The model under review builds one solid part; all positions refer to its coordinate system, in mm. Face numbers are marked on the shaded views. A direction names the side the tool comes from. Give positions to 0.01 mm unless a question says otherwise; leave off trailing zeros. Loops run counter-clockwise (first coordinate to the right, second up) from the corner with the lowest first, then second, coordinate; pieces in that order, holes last. Notation, with made-up numbers: M -13.75,-31.5 L 19.25,-31.5 A25 cw 19.25,-9.5 Z; hole C -17.5,63.25 d3. An arc over 180 degrees is marked long. One line per item, written item: value. Start each with the question number.
Q1. For the marked faces 1 and 2, list the 3-axis set-ups (+Z, -Z, +X, -X, +Y, -Y) from which the entire face can be reached by the end or side of a thin tool; tool diameter is ignored.
Q2. We need section A-A on x = 0. Write out the cut boundary in (y, z), plus the area to 3 significant figures.
Q3. We need section C-C on z = 6.75. Write out the cut boundary in (x, y), plus the area to 3 significant figures.
Q4. To check wall thickness, follow line 1 along Z through (x, y) = (7.5, 1.75); line 2 along Y through (x, z) = (0, 8); line 3 along Y through (x, z) = (3.25, 4.5). State the ranges of each line that lie inside material, in increasing order. Write a range as from..to.
Q5. For pin 1 (1 mm diameter, centred on x = 4, z = 1.5, fed in from -Y); pin 2 (2 mm diameter, centred on y = 7.5, z = 3.5, fed in from +X); pin 3 (4 mm diameter, centred on x = 5.5, y = -6.5, fed in from +Z); pin 4 (6 mm diameter, centred on x = -4.5, y = 2, fed in from +Z), all flat-tipped, find the tip position at first contact; note any pin that passes through.
Q6. We need section D-D on z = 1.75. Write out the cut boundary in (x, y), plus the area to 3 significant figures.
```python
from build123d import *

# Parameters (mm, degrees)
F0_R     = 9.5
F1_DEPTH = 5
F2_R     = 4
F3_DEPTH = 3.5
F4_SIZE  = 1.5
F5_SIZE  = 0.4


with BuildPart() as f1:
    # F0 (on Top) → F1 (new body)
    with BuildSketch(Plane.XY):
        Circle(F0_R)
    extrude(amount=F1_DEPTH)

    # F2 (on face) → F3 (join)
    with BuildSketch(Plane.XY.offset(5)):
        Circle(F2_R)
    extrude(amount=F3_DEPTH)

    # F4
    f4_edges = [f1.edges().sort_by_distance(p)[0] for p in [
        (-9.5, 0, 5),
    ]]
    chamfer(f4_edges, length=F4_SIZE)

    # F5
    f5_edges = [f1.edges().sort_by_distance(p)[0] for p in [
        (-4, 0, 8.5),
    ]]
    chamfer(f5_edges, length=F5_SIZE)


solid = f1.part
```
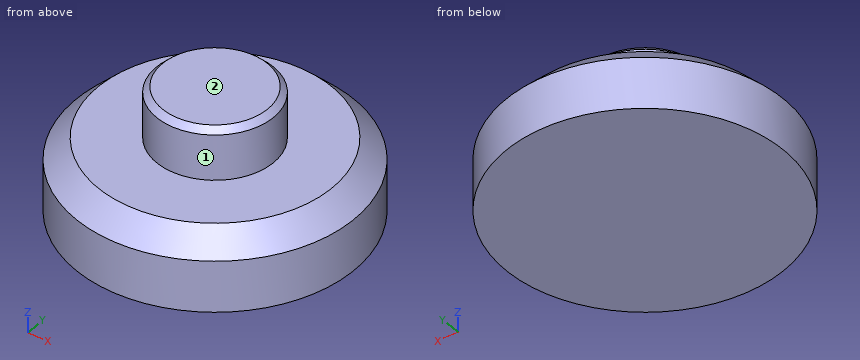
Solved:
1. face 1: +Z
1. face 2: +Z, +X, -X, +Y, -Y
2. outline: M -9.5,0 L 9.5,0 L 9.5,3.5 L 8,5 L 4,5 L 4,8.1 L 3.6,8.5 L -3.6,8.5 L -4,8.1 L -4,5 L -8,5 L -9.5,3.5 Z
2. area: 121 mm2
3. outline: C 0,0 d8
3. area: 50.3 mm2
4. line 1: 0..5
4. line 2: -4..4
4. line 3: -7.85..7.85
5. pin 1: y = -8.83
5. pin 2: x = 6.93
5. pin 3: z = 5
5. pin 4: z = 8.5
6. outline: C 0,0 d19
6. area: 284 mm2
